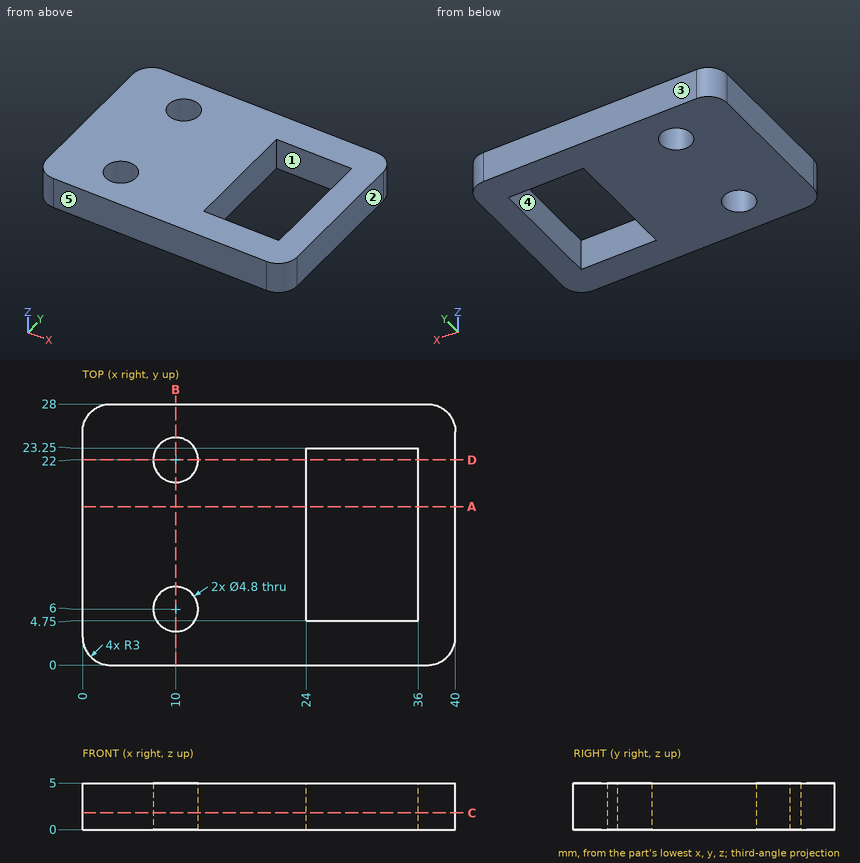
The figure shows three views and two pictorial views of one solid part (mm, origin at its lowest corner). Answer the questions. A direction names the side the tool comes from. Give positions to 0.01 mm unless a question says otherwise; leave off trailing zeros. Write each loop counter-clockwise with the first axis right and the second up, starting at its lowest first coordinate (ties: lowest second). Pieces come first, ordered by that corner, then holes. Notation, with made-up numbers: (70, 39) -> (123, 39) arc R11 ccw to (123, 56) -> close; hole circle Ø7 at (3.5, 38.5). An arc over 180 degrees is marked (long way). Answer as a JSON object with one key per item and string values.
1) A flat-ended cylindrical pin translates along its axis: pin 1 Ø4 at (x, y) = (10, 6) entering from +Z. Find the tip coordinate at first contact, or state that the pin passes through.
Findings below:
{"pin 1": "passes through"}
2) Section D-D on y = 22 is taken. Write down the section's boundary in (x, z), then the cut area to 3 significant figures.
Findings below:
{"outline": "(0, 0) -> (7.6, 0) -> (7.6, 5) -> (0, 5) -> close; (12.4, 0) -> (24, 0) -> (24, 5) -> (12.4, 5) -> close; (36, 0) -> (40, 0) -> (40, 5) -> (36, 5) -> close", "area": "116 mm^2"}
3) Section C-C on z = 1.8 is taken. Write down the section's boundary in (x, y).
Findings below:
{"outline": "(0, 3) arc R3 ccw to (3, 0) -> (37, 0) arc R3 ccw to (40, 3) -> (40, 25) arc R3 ccw to (37, 28) -> (3, 28) arc R3 ccw to (0, 25) -> close; hole circle Ø4.8 at (10, 6); hole circle Ø4.8 at (10, 22); hole (24, 4.75) -> (36, 4.75) -> (36, 23.25) -> (24, 23.25) -> close"}
4) Section A-A on y = 17 is taken. Write down the section's boundary in (x, z), then the cut area to 3 significant figures.
Findings below:
{"outline": "(0, 0) -> (24, 0) -> (24, 5) -> (0, 5) -> close; (36, 0) -> (40, 0) -> (40, 5) -> (36, 5) -> close", "area": "140 mm^2"}
5) Section B-B on x = 10 is taken. Write down the section's boundary in (y, z).
Findings below:
{"outline": "(0, 0) -> (3.6, 0) -> (3.6, 5) -> (0, 5) -> close; (8.4, 0) -> (19.6, 0) -> (19.6, 5) -> (8.4, 5) -> close; (24.4, 0) -> (28, 0) -> (28, 5) -> (24.4, 5) -> close"}
6) Straight lines are drawn through the part: probe 1 along Y at (x, z) = (10, 1.5); probe 2 along X at (y, z) = (18, 4.7); probe 3 along X at (y, z) = (5.5, 1.95). For each, find the intervals that lie inside material, in ascending order. Write a range as from..to.
Findings below:
{"probe 1": "y = 0..3.6, 8.4..19.6, 24.4..28", "probe 2": "x = 0..24, 36..40", "probe 3": "x = 0..7.65, 12.35..24, 36..40"}
7) A tool of negligible diameter and unlimited length cuts with its end or side. For the marked faces 1 and 2, from which of +Z, -Z, +X, -X, +Y, -Y can it reach the whole face along a straight path? Write none if from no direction.
Findings below:
{"face 1": "+Z, -Z", "face 2": "+Z, -Z, +X, +Y, -Y"}
8) For a pull along Y with two mould halves and no side action, classify the marked faces 3, 4 and 5 as pulls with the +Y half, pulls with the -Y half, needs draft (parallel to the pull), parting line crosses it, or undercut.
Findings below:
{"face 3": "pulls with the +Y half", "face 4": "undercut", "face 5": "pulls with the -Y half"}
